Geometry check sheet. Reference: drawing and pictorial views, mm from the part's lowest x, y, z. A direction names the side the tool comes from. Give positions to 0.01 mm unless a question says otherwise; leave off trailing zeros. Order: outer loops, then holes, each group sorted by start corner. A loop starts at its lowest first (then second) coordinate and runs counter-clockwise, first axis right, second up.
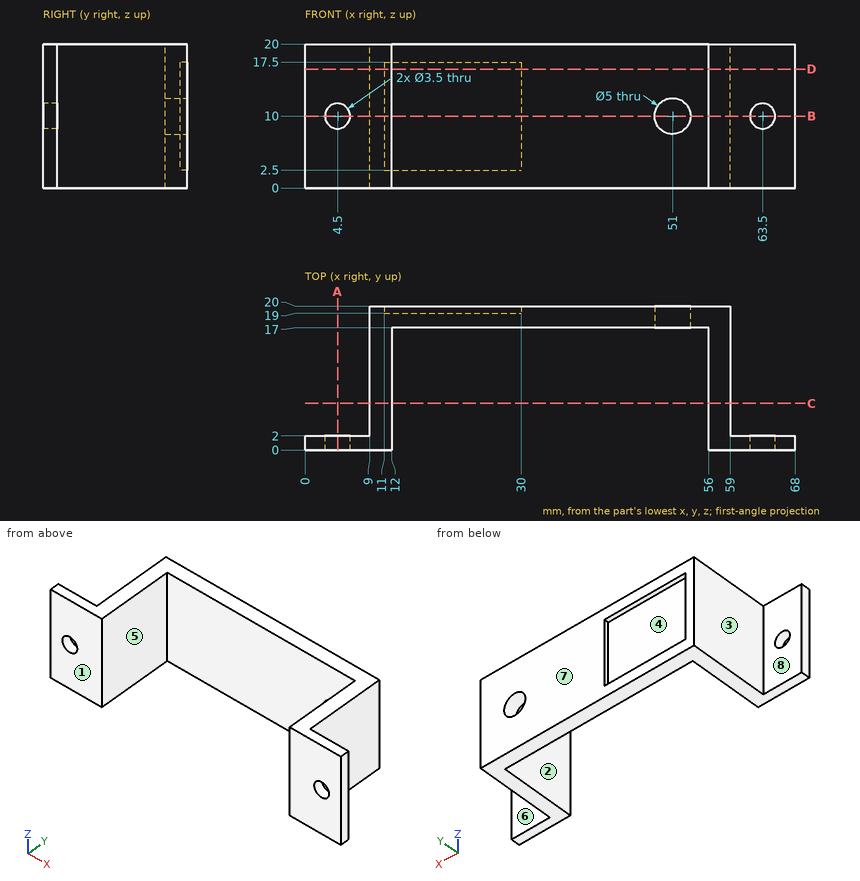
(1) Release check for a two-part mould opening along X. For the marked faces 1, 2 and 3 record: released by +X, released by -X, zero draft, split by the parting line, or undercut.
(2) Sectioned sample at A-A (x = 4.5). Enter the section's corners in (y, z).
(3) Tool access check on the marked faces 4, 5, 6, 7 and 8. Record the directions out of +Z, -Z, +X, -X, +Y, -Y that give a thin tool (end or side, any length) a straight path to the whole face; none if there is none.
(4) Sectioned sample at C-C (y = 6.5). Enter the section's corners in (x, z).
(5) Sectioned sample at D-D (z = 16.5). Enter the section's corners in (x, y), plus the area to 3 significant figures.
(6) Go/stop test with flat-tipped pins: P1, Ø2.5, axis at x = 65.5, z = 8.5, coming from the +Y side; P2, Ø8.5, axis at y = 8.5, z = 14, coming from the -X side; P3, Ø0.8, axis at y = 19.5, z = 7.5, coming from the +X side. Record where each tip stops, or that it passes through.
(7) Thickness scan on L1, parallel to Z at x = 4.5, y = 0.65; L2, parallel to Z at x = 51, y = 19.2; L3, parallel to X at y = 9.75, z = 17.5. Record the ranges inside material, lowest first.
(8) Sectioned sample at B-B (z = 10). Enter the section's corners in (x, y), plus the area to 3 significant figures.
Values follow:
1. face 1: zero draft
1. face 2: undercut
1. face 3: released by -X
2. outline: (0, 0) - (2, 0) - (2, 8.25) - (0, 8.25) - close; (0, 11.75) - (2, 11.75) - (2, 20) - (0, 20) - close
3. face 4: +Y
3. face 5: +Z, -Z, -Y
3. face 6: +Z, -Z, +X, +Y
3. face 7: +Z, -Z, +X, -X, +Y
3. face 8: +Z, -Z, -X, +Y
4. outline: (9, 0) - (12, 0) - (12, 20) - (9, 20) - close; (56, 0) - (59, 0) - (59, 20) - (56, 20) - close
5. outline: (0, 0) - (12, 0) - (12, 17) - (56, 17) - (56, 0) - (68, 0) - (68, 2) - (59, 2) - (59, 20) - (30, 20) - (30, 19) - (11, 19) - (11, 20) - (9, 20) - (9, 2) - (0, 2) - close
5. area: 269 mm2
6. P1: stops at y = 2
6. P2: stops at x = 9
6. P3: stops at x = 59
7. L1: z = 0 to 8.25, 11.75 to 20
7. L2: z = 0 to 7.5, 12.5 to 20
7. L3: x = 9 to 12, 56 to 59
8. outline: (0, 0) - (2.75, 0) - (2.75, 2) - (0, 2) - close; (6.25, 0) - (12, 0) - (12, 17) - (48.5, 17) - (48.5, 20) - (30, 20) - (30, 19) - (11, 19) - (11, 20) - (9, 20) - (9, 2) - (6.25, 2) - close; (53.5, 17) - (56, 17) - (56, 0) - (61.75, 0) - (61.75, 2) - (59, 2) - (59, 20) - (53.5, 20) - close; (65.25, 0) - (68, 0) - (68, 2) - (65.25, 2) - close
8. area: 240 mm2
